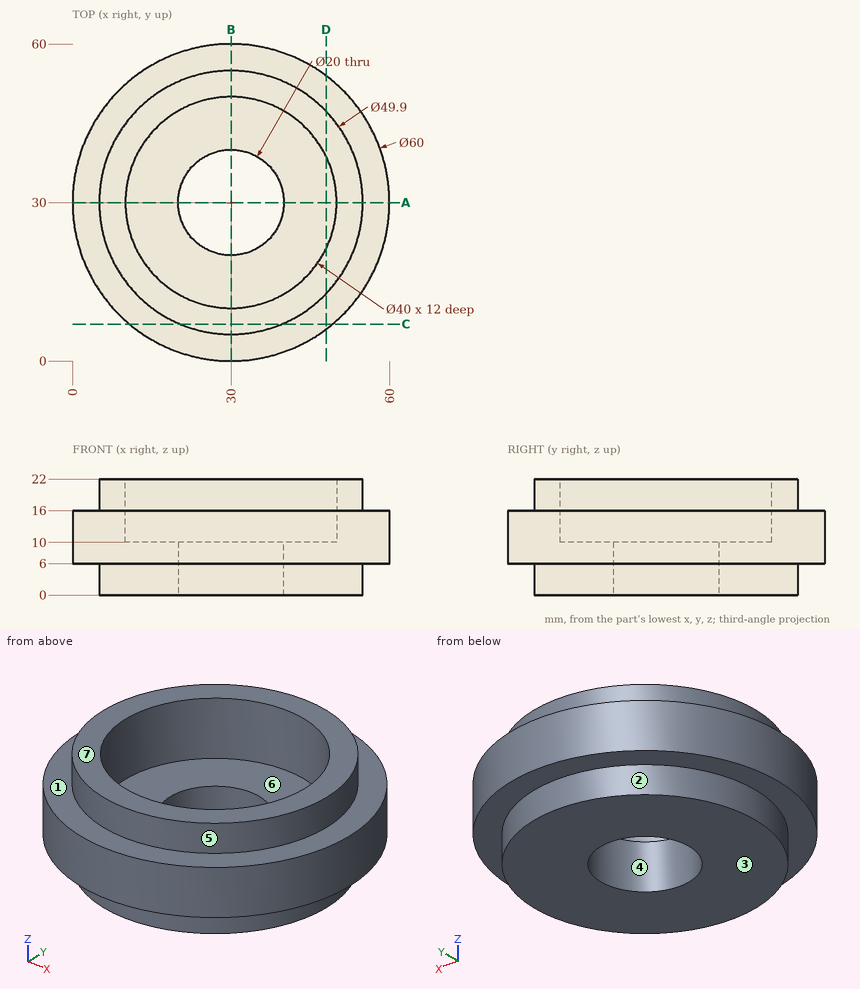
Geometry: see drawing. Coordinates: mm, zero at the bounding-box minimum. A direction names the side the tool comes from. Round coordinates to 2 decimals unless told otherwise and drop trailing zeros. Write each loop counter-clockwise with the first axis right and the second up, starting at its lowest first coordinate (ties: lowest second). Pieces come first, ordered by that corner, then holes.
Item 1: Pin query (flat end, axial travel): P1, Ø1.5, axis at x = 24.5, z = 10.5, coming from the -Y side; P2, Ø1.5, axis at x = 10.5, z = 18.5, coming from the -Y side; P3, Ø24, axis at x = 30, y = 30, coming from the +Z side. Return the tip coordinate at first contact, or that it passes through.
Item 2: Section query A-A (y = 30). Return loops of the section in (x, z), plus the area to 3 significant figures.
Item 3: Material intervals for L1, parallel to Y at x = 30, z = 3; L2, parallel to X at y = 29.5, z = 8.25; L3, parallel to Z at x = 30.5, y = 40.5, sorted ascending.
Item 4: Section query C-C (y = 7). Return loops of the section in (x, z).
Item 5: Section query D-D (x = 48). Return loops of the section in (y, z), plus the area to 3 significant figures.
Item 6: Mould query, pull axis Y, two halves, no side actions, for the marked faces 4, 5, 6 and 7. Classes: +Y half, -Y half, draft (parallel to the pull), parting line (faces both ways), or undercut.
Item 7: Set-up query: the marked faces 1, 2 and 3. Return all of +Z, -Z, +X, -X, +Y, -Y with unobstructed straight access to the full face (end or side cutting, diameter ignored); none if empty.
Completed:
1. P1: stops at y = 0.38
1. P2: stops at y = 13.54
1. P3: stops at z = 10
2. outline: (0, 6) - (5.05, 6) - (5.05, 0) - (20, 0) - (20, 10) - (10, 10) - (10, 22) - (5.05, 22) - (5.05, 16) - (0, 16) - close; (40, 0) - (54.95, 0) - (54.95, 6) - (60, 6) - (60, 16) - (54.95, 16) - (54.95, 22) - (50, 22) - (50, 10) - (40, 10) - close
2. area: 519 mm2
3. L1: y = 5.05 to 20, 40 to 54.95
3. L2: x = 0 to 20.01, 39.99 to 60
3. L3: z = 0 to 10
4. outline: (10.74, 6) - (20.33, 6) - (20.33, 0) - (39.67, 0) - (39.67, 6) - (49.26, 6) - (49.26, 16) - (39.67, 16) - (39.67, 22) - (20.33, 22) - (20.33, 16) - (10.74, 16) - close
5. outline: (6, 6) - (12.72, 6) - (12.72, 0) - (47.28, 0) - (47.28, 6) - (54, 6) - (54, 16) - (47.28, 16) - (47.28, 22) - (38.72, 22) - (38.72, 10) - (21.28, 10) - (21.28, 22) - (12.72, 22) - (12.72, 16) - (6, 16) - close
5. area: 685 mm2
6. face 4: undercut
6. face 5: parting line
6. face 6: undercut
6. face 7: draft
7. face 1: +Z
7. face 2: -Z
7. face 3: -Z, +X, -X, +Y, -Y
